CAD build for the part. Positions are in the model's coordinates, mm. Face numbers are marked on the shaded views. A direction names the side the tool comes from. Coordinates: 2 decimals unless noted, no trailing zeros. Loops run counter-clockwise (first coordinate to the right, second up) from the corner with the lowest first, then second, coordinate; pieces in that order, holes last.
1) Which spindle directions (+Z, -Z, +X, -X, +Y, -Y) get a long thin tool onto all of the face, cutting with end or side? Do the marked faces 1, 2, 3, 4 and 5. Say none if no direction does.
2) Saw through at C-C, the plane y = 15. Write the cut outline in (x, z).
3) Saw through at D-D, the plane x = 0. Write the cut outline in (y, z), and give its area (3 significant figures).
4) Two-plate mould, pull along Z, no slides. Class the marked faces 6, 7 and 8: +Z half, -Z half, draft (parallel to the pull), parting line (faces both ways), or undercut.
5) Saw through at A-A, the plane z = -10. Write the cut outline in (x, y).
6) Saw through at B-B, the plane x = -22. Write the cut outline in (y, z), and give its area (3 significant figures).
7) Pin check, flat tips, straight feed: pin 1 Ø3 at (x, y) = (9, 58) entering from +Z; pin 2 Ø4 at (x, z) = (0, 70) entering from -Y; pin 3 Ø9 at (x, y) = (16.5, 11) entering from -Z. Stop position of each tip, or through.
8) Wall check: line 1 along Z through (x, y) = (-5, 2); line 2 along X through (y, z) = (3.5, -10); line 3 along X through (y, z) = (4, 70). Give the ranges that are in metal, low to high.
```python
from build123d import *
from OCP.BRepFilletAPI import BRepFilletAPI_MakeChamfer

# Parameters (mm, degrees)
SKETCH1_W           = 15
SKETCH1_H           = 27.5
SKETCH1_W_2         = 10
SKETCH1_H_2         = 20
BOSS_EXTRUDE1_DEPTH = 5
SKETCH8_W           = 15
SKETCH8_H           = 90
BOSS_EXTRUDE2_DEPTH = 5
SKETCH9_R           = 2.6
CUT_EXTRUDE1_DEPTH  = 11
SKETCH11_W          = 50
SKETCH11_H          = 15
BOSS_EXTRUDE4_DEPTH = 15
CHAMFER1_SIZE       = 5
CHAMFER1_SIZE_2     = 17.437072219
CHAMFER2_SIZE       = 15.722257417
CHAMFER2_SIZE_2     = 7
SKETCH12_R          = 2
CUT_EXTRUDE2_DEPTH  = 122.783619588
SKETCH13_W          = 15
SKETCH13_H          = 10
BOSS_EXTRUDE5_DEPTH = 5
SKETCH15_W          = 5
SKETCH15_H          = 35
BOSS_EXTRUDE7_DEPTH = 5
BOSS_EXTRUDE8_DEPTH = 5
FILLET1_R           = 15
FILLET2_R           = 20
CHAMFER3_SIZE       = 17.5


# Read off the part's stored shape, not the designer's step: Ø3.0mm Dowel Hole1
# Some blends are built 0.0001 mm under size
with BuildPart() as part:
    # Sketch1 → Boss-Extrude1 (new body)
    # profile 1 of 2: a face of its own
    with BuildSketch(Plane(origin=(0, 0, 0), x_dir=(1, 0, 0), z_dir=(0, 1, 0))):
        with Locations((0, -1.25)):
            Rectangle(SKETCH1_W, SKETCH1_H)
        Rectangle(SKETCH1_W_2, SKETCH1_H_2, mode=Mode.SUBTRACT)
    # profile 2 of 2: a face of its own
    with BuildSketch(Plane(origin=(0, 0, 0), x_dir=(1, 0, 0), z_dir=(0, 1, 0))):
        Rectangle(SKETCH1_W_2, SKETCH1_H_2)
    extrude(amount=BOSS_EXTRUDE1_DEPTH)

    # Ø3.0mm Dowel Hole1 outline → Ø3.0mm Dowel Hole1 (revolve, cut)
    with BuildSketch(Plane(origin=(5, 0, -10), x_dir=(1, 0, 0), z_dir=(0, 0, 1))):
        Polygon((0, 0), (1.6, 0), (1.6, 4.874135055), (1.75, 5), (0, 5), align=None)
    revolve(axis=Axis((5, 0, -10), (0, 1, 0)), mode=Mode.SUBTRACT)

    # 3.0mm Dowel Hole1 2 outline → 3.0mm Dowel Hole1 2 (revolve, cut)
    with BuildSketch(Plane(origin=(-5, 0, 10), x_dir=(1, 0, 0), z_dir=(0, 0, 1))):
        Polygon((0, 0), (1.6, 0), (1.6, 4.874135055), (1.75, 5), (0, 5), align=None)
    revolve(axis=Axis((-5, 0, 10), (0, 1, 0)), mode=Mode.SUBTRACT)

    # 3.0mm Dowel Hole1 3 outline → 3.0mm Dowel Hole1 3 (revolve, cut)
    with BuildSketch(Plane(origin=(-5, 0, -10), x_dir=(1, 0, 0), z_dir=(0, 0, 1))):
        Polygon((0, 0), (1.6, 0), (1.6, 4.874135055), (1.75, 5), (0, 5), align=None)
    revolve(axis=Axis((-5, 0, -10), (0, 1, 0)), mode=Mode.SUBTRACT)

    # 3.0mm Dowel Hole1 4 outline → 3.0mm Dowel Hole1 4 (revolve, cut)
    with BuildSketch(Plane(origin=(5, 0, 10), x_dir=(1, 0, 0), z_dir=(0, 0, 1))):
        Polygon((0, 0), (1.6, 0), (1.6, 4.874135055), (1.75, 5), (0, 5), align=None)
    revolve(axis=Axis((5, 0, 10), (0, 1, 0)), mode=Mode.SUBTRACT)

    # Sketch8 → Boss-Extrude2 (add)
    with BuildSketch(Plane(origin=(0, 5, 0), x_dir=(1, 0, 0), z_dir=(0, 1, 0))):
        with Locations((0, -60)):
            Rectangle(SKETCH8_W, SKETCH8_H)
    extrude(amount=-BOSS_EXTRUDE2_DEPTH)

    # Sketch9 → Cut-Extrude1 (cut)
    with BuildSketch(Plane(origin=(0, 0, 0), x_dir=(1, 0, 0), z_dir=(0, 1, 0))):
        with Locations(Location((0, -70, 0), (0, 0, 270))):
            Circle(SKETCH9_R)
    extrude(amount=CUT_EXTRUDE1_DEPTH, mode=Mode.SUBTRACT)

    # Sketch11 → Boss-Extrude4 (add)
    with BuildSketch(Plane(origin=(0, 5, 0), x_dir=(1, 0, 0), z_dir=(0, 1, 0))):
        with Locations((0, -97.5)):
            Rectangle(SKETCH11_W, SKETCH11_H)
    extrude(amount=BOSS_EXTRUDE4_DEPTH)

    # Chamfer1
    chamfer1_edges_1 = [part.edges().sort_by_distance(p)[0] for p in [
        (7.5, 5, 97.5),
    ]]
    chamfer1_side_1 = [part.faces().sort_by_distance(p)[0] for p in [
        (7.5, 4.9, 97.5),
    ]]
    chamfer1_edges_2 = [part.edges().sort_by_distance(p)[0] for p in [
        (-7.5, 5, 97.5),
    ]]
    chamfer1_side_2 = [part.faces().sort_by_distance(p)[0] for p in [
        (-7.5, 4.9, 97.5),
    ]]
    chamfer1 = BRepFilletAPI_MakeChamfer(part.part.solid().wrapped)
    for e in chamfer1_edges_1:
        chamfer1.Add(CHAMFER1_SIZE - 0.0001, CHAMFER1_SIZE_2 - 0.0001, e.wrapped, chamfer1_side_1[0].wrapped)
    for e in chamfer1_edges_2:
        chamfer1.Add(CHAMFER1_SIZE - 0.0001, CHAMFER1_SIZE_2 - 0.0001, e.wrapped, chamfer1_side_2[0].wrapped)
    add(Compound.cast(chamfer1.Shape()), mode=Mode.REPLACE)  # a hair under: the kernel refuses the full size

    # Chamfer2
    # the kernel refuses this chamfer: 15.722257417, 7 mm, written as the material it adds along each edge
    with BuildSketch(Plane(origin=(-7.5, 5, 90), x_dir=(0, 0.9998768419809391, 0.015693975602887097), z_dir=(1, 0, 0))) as chamfer2_piece_1_section:
        Polygon((CHAMFER2_SIZE * 0.999876842002, -CHAMFER2_SIZE * 0.0156939756032), (-CHAMFER2_SIZE_2 * 0.0156939756029, -CHAMFER2_SIZE_2 * 0.999876841981), (0, 0), align=None)
    chamfer2_piece_1 = extrude(amount=15, mode=Mode.PRIVATE)
    chamfer2_piece_1 = split(chamfer2_piece_1, bisect_by=Plane(origin=(0, 20, 87.661958793), z_dir=(0, -1, 0)), keep=Keep.TOP, mode=Mode.PRIVATE)
    add(chamfer2_piece_1)

    # Sketch12 → Cut-Extrude2 (cut, through all)
    with BuildSketch(Plane.XY.offset(105)):
        with Locations((-18, 15)):
            Circle(SKETCH12_R)
        with Locations((18, 15)):
            Circle(SKETCH12_R)
    extrude(amount=-CUT_EXTRUDE2_DEPTH, mode=Mode.SUBTRACT)

    # Sketch13 → Boss-Extrude5 (add)
    with BuildSketch(Plane(origin=(0, 5, 0), x_dir=(1, 0, 0), z_dir=(0, 1, 0))):
        with Locations((0, 17.5)):
            Rectangle(SKETCH13_W, SKETCH13_H)
    extrude(amount=-BOSS_EXTRUDE5_DEPTH)

    # Sketch15 → Boss-Extrude7 (add)
    with BuildSketch(Plane(origin=(0, 5, 0), x_dir=(1, 0, 0), z_dir=(0, 1, 0))):
        with Locations((-22.5, 40)):
            Rectangle(SKETCH15_W, SKETCH15_H)
        Polygon((-7.5, 17.5), (-7.5, 22.5), (-20, 22.5), (-25, 22.5), (-25, 17.5), align=None)
        Polygon((25, 17.5), (25, 22.5), (20, 22.5), (7.5, 22.5), (7.5, 17.5), align=None)
        with Locations((22.5, 40)):
            Rectangle(SKETCH15_W, SKETCH15_H)
    extrude(amount=-BOSS_EXTRUDE7_DEPTH)

    # Sketch16 → Boss-Extrude8 (add)
    with BuildSketch(Plane(origin=(0, 0, -57.5), x_dir=(-1, 0, 0), z_dir=(0, 0, -1))):
        with BuildLine():
            Line((-20, 40), (-25, 40))
            ThreePointArc((-25, 40), (-23.717082451, 32.09430585), (-20, 25))
            Line((-20, 25), (-20, 40))
        make_face()
        with BuildLine():
            Line((20, 40), (25, 40))
            ThreePointArc((25, 40), (0, 65), (-25, 40))
            Line((-25, 40), (-20, 40))
            ThreePointArc((-20, 40), (0, 60), (20, 40))
        make_face()
        with BuildLine():
            ThreePointArc((20, 25), (23.717082451, 32.09430585), (25, 40))
            Line((25, 40), (20, 40))
            Line((20, 40), (20, 25))
        make_face()
        with BuildLine():
            Line((20, 5), (25, 5))
            Line((25, 5), (25, 40))
            ThreePointArc((25, 40), (23.717082451, 32.09430585), (20, 25))
            Line((20, 25), (20, 5))
        make_face()
        with BuildLine():
            ThreePointArc((-20, 25), (-23.717082451, 32.09430585), (-25, 40))
            Line((-25, 40), (-25, 0))
            Line((-25, 0), (-20, 0))
            Line((-20, 0), (-20, 25))
        make_face()
    extrude(amount=-BOSS_EXTRUDE8_DEPTH)

    # Fillet1
    fillet1_edges = [part.edges().sort_by_distance(p)[0] for p in [
        (-22.5, 5, -52.5),
        (22.5, 5, -52.5),
    ]]
    fillet(fillet1_edges, radius=FILLET1_R)

    # Fillet2
    fillet2_edges = [part.edges().sort_by_distance(p)[0] for p in [
        (-22.5, 0, -57.5),
        (22.5, 0, -57.5),
    ]]
    fillet(fillet2_edges, radius=FILLET2_R)

    # Chamfer3
    chamfer3_edges = [part.edges().sort_by_distance(p)[0] for p in [
        (-25, 2.5, -17.5),
        (-20, 2.5, -22.5),
        (25, 2.5, -17.5),
        (20, 2.5, -22.5),
    ]]
    chamfer(chamfer3_edges, length=CHAMFER3_SIZE - 0.0001)  # a hair under: the kernel refuses the full size


solid = part.part
```
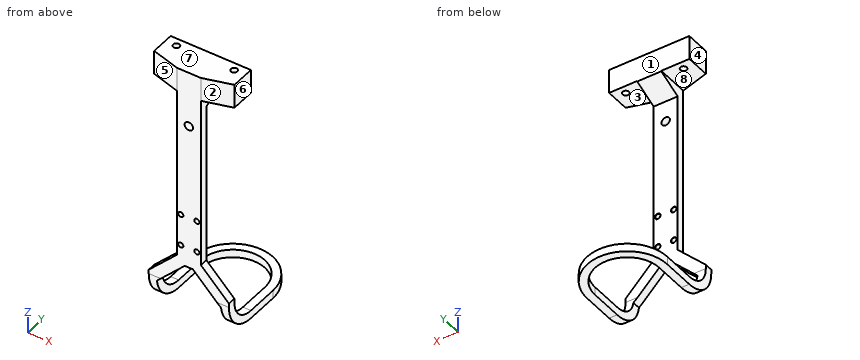
Data:
1. face 1: +Z, +X, -X, +Y
1. face 2: +Z, +X, -Y
1. face 3: +X, +Y, -Y
1. face 4: +Z, -Z, -X, +Y, -Y
1. face 5: +Z, -X, -Y
2. outline: (-25, -56.86) - (-20, -56.86) - (-20, -51.64) - (-25, -51.64) - close; (-25, 90) - (-20, 90) - (-20, 105) - (-25, 105) - close; (-16, 90) - (-7.5, 90) - (-7.5, 87.45) - (7.5, 87.45) - (7.5, 90) - (16, 90) - (16, 105) - (-16, 105) - close; (20, -56.86) - (25, -56.86) - (25, -51.64) - (20, -51.64) - close; (20, 90) - (25, 90) - (25, 105) - (20, 105) - close
3. outline: (0, -22.5) - (5, -22.5) - (5, 67.4) - (0, 67.4) - close; (0, 72.6) - (5, 72.6) - (5, 83) - (20, 89.68) - (20, 105) - (0, 105) - close; (60, -57.5) - (65, -57.5) - (65, -52.5) - (60, -52.5) - close
3. area: 916 mm2
4. face 6: draft
4. face 7: +Z half
4. face 8: undercut
5. outline: (-7.5, 0) - (-6.6, 0) - (-6.6, 4.87) - (-6.75, 5) - (-7.5, 5) - close; (-3.4, 0) - (3.4, 0) - (3.4, 4.87) - (3.25, 5) - (-3.25, 5) - (-3.4, 4.87) - close; (6.6, 0) - (7.5, 0) - (7.5, 5) - (6.75, 5) - (6.6, 4.87) - close
6. outline: (0, -37.5) arc R20 ccw to (20, -57.5) - (51.87, -57.5) - (51.87, -52.5) - (20, -52.5) arc R15 cw to (5, -37.5) - (5, -32) - (0, -32) - close; (4.16, 90) - (20, 90) - (20, 105) - (4.16, 105) - close
6. area: 562 mm2
7. pin 1: stops at z = -52.5
7. pin 2: passes through
7. pin 3: stops at z = -56.52
8. line 1: z = -25 to -11.6, -8.4 to 8.4, 11.6 to 105
8. line 2: x = -7.5 to -6.6, -3.4 to 3.4, 6.6 to 7.5
8. line 3: x = -7.5 to -2.6, 2.6 to 7.5
